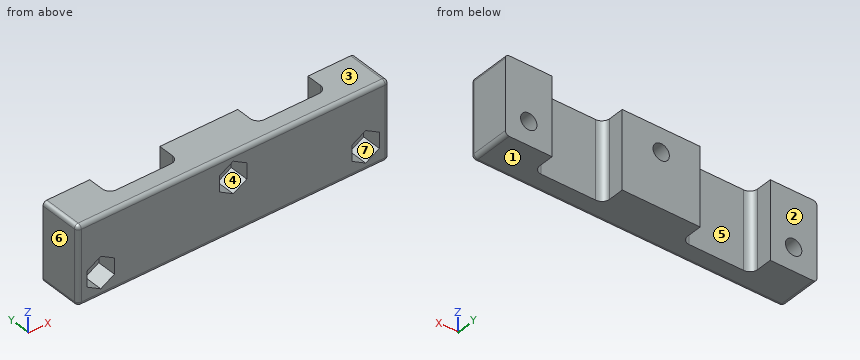
```python
from build123d import *

# Parameters (mm, degrees)
SKETCH_W        = 80
SKETCH_H        = 20
PAD_DEPTH       = 11
SKETCH001_R     = 2.1
POCKET_DEPTH    = 11.001
POCKET001_DEPTH = 5
SKETCH003_W     = 18
SKETCH003_H     = 6
POCKET002_DEPTH = 20.001
FILLET_R        = 2
FILLET001_R     = 2
FILLET002_R     = 2
FILLET003_R     = 2
FILLET004_R     = 1


with BuildPart() as part:
    # Sketch → Pad (new body)
    with BuildSketch(Plane.XZ):
        with Locations((40, 10)):
            Rectangle(SKETCH_W, SKETCH_H)
    extrude(amount=PAD_DEPTH)

    # Sketch001 (on Face6 of Pad) → Pocket (cut, through all)
    with BuildSketch(Plane.XZ.offset(11)):
        with Locations((6, 6)):
            Circle(SKETCH001_R)
        with Locations((40, 14)):
            Circle(SKETCH001_R)
        with Locations((74, 6)):
            Circle(SKETCH001_R)
    extrude(amount=-POCKET_DEPTH, mode=Mode.SUBTRACT)

    # Sketch002 (on Face5 of Pocket) → Pocket001 (cut)
    with BuildSketch(Plane.XZ.offset(11)):
        Polygon((9.5, 3.979274), (9.5, 8.020726), (6, 10.041452), (2.5, 8.020726), (2.5, 3.979274), (6, 1.958548), align=None)
        Polygon((40, 9.958548), (43.5, 11.979274), (43.5, 16.020726), (40, 18.041452), (36.5, 16.020726), (36.5, 11.979274), align=None)
        Polygon((77.5, 3.979274), (77.5, 8.020726), (74, 10.041452), (70.5, 8.020726), (70.5, 3.979274), (74, 1.958548), align=None)
    extrude(amount=-POCKET001_DEPTH, mode=Mode.SUBTRACT)

    # Sketch003 (on Face6 of Pocket001) → Pocket002 (cut, through all)
    with BuildSketch(Plane(origin=(0, 0, 20), x_dir=(-1, 0, 0), z_dir=(0, 0, 1))):
        with Locations((-59, 3)):
            Rectangle(SKETCH003_W, SKETCH003_H)
        with Locations((-21, 3)):
            Rectangle(SKETCH003_W, SKETCH003_H)
    extrude(amount=-POCKET002_DEPTH, mode=Mode.SUBTRACT)

    # Fillet
    fillet_edges = [part.edges().sort_by_distance(p)[0] for p in [
        (50, -6, 10),
    ]]
    fillet(fillet_edges, radius=FILLET_R)

    # Fillet001
    fillet001_edges = [part.edges().sort_by_distance(p)[0] for p in [
        (12, -6, 10),
    ]]
    fillet(fillet001_edges, radius=FILLET001_R)

    # Fillet002
    fillet002_edges = [part.edges().sort_by_distance(p)[0] for p in [
        (30, -6, 10),
    ]]
    fillet(fillet002_edges, radius=FILLET002_R)

    # Fillet003
    fillet003_edges = [part.edges().sort_by_distance(p)[0] for p in [
        (68, -6, 10),
    ]]
    fillet(fillet003_edges, radius=FILLET003_R)

    # Fillet004
    fillet004_edges = [part.edges().sort_by_distance(p)[0] for p in [
        (0, -5.5, 0),
        (40, -11, 0),
        (0, -11, 10),
        (40, -11, 20),
        (80, -11, 10),
        (80, -5.5, 0),
        (80, -5.5, 20),
        (0, -5.5, 20),
    ]]
    fillet(fillet004_edges, radius=FILLET004_R)


solid = part.part
```
Input: part model. Units: mm. Frame: model coordinates. Face numbers are marked on the shaded views. A direction names the side the tool comes from. Give positions to 0.01 mm unless a question says otherwise; leave off trailing zeros. Order: outer loops, then holes, each group sorted by start corner. A loop starts at its lowest first (then second) coordinate and runs counter-clockwise, first axis right, second up.
1. Pin query (flat end, axial travel): pin 1 Ø3.5 at (x, z) = (39.5, 12.5) entering from -Y; pin 2 Ø1.5 at (x, z) = (56, 14.5) entering from +Y; pin 3 Ø1.5 at (x, y) = (36.5, -2.5) entering from -Z. Return the tip coordinate at first contact, or that it passes through.
Computed:
pin 1: stops at y = -6
pin 2: stops at y = -6
pin 3: stops at z = 0
2. Cut plane D-D (z = 6). State how many separate pieces and enclosed holes the cut face has, and give its area (3 significant figures).
Computed:
separate pieces: 3
enclosed holes: 0
area: 547 mm2
3. Draft query along Z for the marked faces 1, 2, 3 and 4. Return one class per face: released by +Z, released by -Z, zero draft, split by the parting line, or undercut.
Computed:
face 1: released by -Z
face 2: zero draft
face 3: released by +Z
face 4: undercut
4. Cut plane B-B (z = 14). Return loops of the section in (x, y).
Computed:
outline: (0, -10) arc R1 ccw to (1, -11) - (36.5, -11) - (36.5, -6) - (37.9, -6) - (37.9, 0) - (30, 0) - (30, -4) arc R2 cw to (28, -6) - (14, -6) arc R2 cw to (12, -4) - (12, 0) - (0, 0) - close; (42.1, -6) - (43.5, -6) - (43.5, -11) - (79, -11) arc R1 ccw to (80, -10) - (80, 0) - (68, 0) - (68, -4) arc R2 cw to (66, -6) - (52, -6) arc R2 cw to (50, -4) - (50, 0) - (42.1, 0) - close
5. Set-up query: the marked faces 5, 6 and 7. Return all of +Z, -Z, +X, -X, +Y, -Y with unobstructed straight access to the full face (end or side cutting, diameter ignored); none if empty.
Computed:
face 5: +Z, -Z, +Y
face 6: +Z, -Z, -X, +Y, -Y
face 7: -Y
6. Line query: probe 1 along X at (y, z) = (-3, 2); probe 2 along X at (y, z) = (-8.5, 4); probe 3 along Z at (x, y) = (74, -2.5). Output: solid intervals per line, ascending.
Computed:
probe 1: x = 0 to 12, 30 to 50, 68 to 80
probe 2: x = 0 to 2.5, 9.5 to 70.5, 77.5 to 80
probe 3: z = 0 to 3.9, 8.1 to 20
7. Cut plane C-C (y = -7.75). Return loops of the section in (x, z), and give its area (3 significant figures).
Computed:
outline: (0, 1) arc R1 ccw to (1, 0) - (79, 0) arc R1 ccw to (80, 1) - (80, 19) arc R1 ccw to (79, 20) - (1, 20) arc R1 ccw to (0, 19) - close; hole (2.5, 3.98) - (6, 1.96) - (9.5, 3.98) - (9.5, 8.02) - (6, 10.04) - (2.5, 8.02) - close; hole (36.5, 11.98) - (40, 9.96) - (43.5, 11.98) - (43.5, 16.02) - (40, 18.04) - (36.5, 16.02) - close; hole (70.5, 3.98) - (74, 1.96) - (77.5, 3.98) - (77.5, 8.02) - (74, 10.04) - (70.5, 8.02) - close
area: 1,470 mm2
8. Cut plane A-A (y = -2.25). Return loops of the section in (x, z), and give its area (3 significant figures).
Computed:
outline: (0, 1) arc R1 ccw to (1, 0) - (12, 0) - (12, 20) - (1, 20) arc R1 ccw to (0, 19) - close; (30, 0) - (50, 0) - (50, 20) - (30, 20) - close; (68, 0) - (79, 0) arc R1 ccw to (80, 1) - (80, 19) arc R1 ccw to (79, 20) - (68, 20) - close; hole circle Ø4.2 at (6, 6); hole circle Ø4.2 at (40, 14); hole circle Ø4.2 at (74, 6)
area: 838 mm2
